from build123d import *

# Parameters (mm, degrees)
SKETCH1_R                   = 5.5
SKETCH1_W                   = 4
SKETCH1_H                   = 2
BOSS_EXTRUDE1_DEPTH         = 5
SKETCH2_R                   = 11.5
BOSS_EXTRUDE2_DEPTH         = 3
SKETCH3_R                   = 1.5
WHEEL_SCREWS_DEPTH          = 3
WHEEL_SCREW_PATTERN_COUNT   = 3
SKETCH5_R                   = 0.95
MOTOR_SCREW_HOLE_DEPTH      = 3
MOTOR_SCREW_HOLE_DEPTH_BACK = 8.474829283


with BuildPart() as part:
    # Sketch1 → Boss-Extrude1 (new body)
    with BuildSketch(Plane(origin=(0, 0, 0), x_dir=(1, 0, 0), z_dir=(0, 1, 0))):
        Circle(SKETCH1_R)
        with BuildLine():
            Line((-1.095, -1.025170717), (1.095, -1.025170717))
            ThreePointArc((1.095, -1.025170717), (0, 1.5), (-1.095, -1.025170717))
        make_face(mode=Mode.SUBTRACT)
        with Locations((0, -3.025170717)):
            Rectangle(SKETCH1_W, SKETCH1_H, mode=Mode.SUBTRACT)
    extrude(amount=BOSS_EXTRUDE1_DEPTH)

    # Sketch2 → Boss-Extrude2 (add)
    with BuildSketch(Plane(origin=(0, 5, 0), x_dir=(1, 0, 0), z_dir=(0, 1, 0))):
        Circle(SKETCH2_R)
    extrude(amount=BOSS_EXTRUDE2_DEPTH)

    # Sketch3 → wheel_screws (cut)
    with BuildSketch(Plane.XZ.offset(-5)):
        with Locations((0, -8.5)):
            Circle(SKETCH3_R)
    wheel_screws = extrude(amount=-WHEEL_SCREWS_DEPTH, mode=Mode.SUBTRACT)

    # wheel_screw_pattern: wheel_screws ×3 about axis
    wheel_screw_pattern_axis = Axis((0, 0, 0), (0, 1, 0))
    for i in range(1, WHEEL_SCREW_PATTERN_COUNT):
        add(wheel_screws.rotate(wheel_screw_pattern_axis, i * 360 / WHEEL_SCREW_PATTERN_COUNT), mode=Mode.SUBTRACT)

    # Sketch5 → motor_screw_hole (cut, two sides)
    with BuildSketch(Plane(origin=(0, 0, 4.025170717), x_dir=(-1, 0, 0), z_dir=(0, 0, -1))) as motor_screw_hole_sk:
        with Locations((0, 2.5)):
            Circle(SKETCH5_R)
    extrude(amount=MOTOR_SCREW_HOLE_DEPTH, mode=Mode.SUBTRACT)
    extrude(motor_screw_hole_sk.sketch, amount=-MOTOR_SCREW_HOLE_DEPTH_BACK, mode=Mode.SUBTRACT)


solid = part.part
Here's how the part is built. I have some questions about the finished solid (model axes, mm). A direction names the side the tool comes from. Coordinates: 2 decimals unless noted, no trailing zeros. Write each loop counter-clockwise with the first axis right and the second up, starting at its lowest first coordinate (ties: lowest second). Pieces come first, ordered by that corner, then holes.
Item 1: I want a section at D-D on z = 3.25. Write out the boundary of the cut face in (x, y).
Item 2: I want a section at A-A on z = 0. Write out the boundary of the cut face in (x, y).
Item 3: If I drill on line 1 (Z direction, x = 0, y = 3.7); line 2 (Z direction, x = 0, y = 7.2); line 3 (X direction, y = 6, z = 4.5), over which ranges is the centre line in solid material (lowest first)?
Item 4: Will these pins go through, and if not, where does the flat tip stop? pin 1 (1.6 mm diameter, centred on y = 3.5, z = 3, fed in from -X); pin 2 (2.5 mm diameter, centred on x = 0, y = 2.5, fed in from +Z); pin 3 (2 mm diameter, centred on y = 6, z = 9, fed in from +X).
Item 5: I want a section at B-B on x = 0. Write out the boundary of the cut face in (y, z), and give its area (3 significant figures).
Item 6: If we mould it in two halves opening along Z, with no side actions, what happens to faces 4 (the cylindrical face through (0, 6, -10)), 5 (the cylindrical face through (-1.5, 6.5, -11.4)), 6 (the flat face through (5, 5, -3))? For each: +Z half, -Z half, draft (parallel to the pull), parting line (faces both ways), or undercut.
Item 7: I want a section at C-C on x = -6.75. Write out the boundary of the cut face in (y, z).
Item 8: On a 3-axis mill with a long thin cutter (end or side, diameter ignored), from which of +Z, -Z, +X, -X, +Y, -Y can I reach the whole of each face in a straight line? I mean faces 1 (the flat face through (-1, 2, 2.025)), 2 (the flat face through (1.1, 0, -1.3)), 3 (the cylindrical face through (0.124, 3.442, 4.752)). Say none if no direction works.
Findings below:
1. outline: (-11.03, 5) - (-8.48, 5) - (-8.48, 8) - (-11.03, 8) - close; (-6.24, 5) - (-4.44, 5) - (-4.44, 0) - (-2, 0) - (-2, 5) - (2, 5) - (2, 0) - (4.44, 0) - (4.44, 5) - (6.24, 5) - (6.24, 8) - (-6.24, 8) - close; (8.48, 5) - (11.03, 5) - (11.03, 8) - (8.48, 8) - close
2. outline: (-11.5, 5) - (-5.5, 5) - (-5.5, 0) - (-1.5, 0) - (-1.5, 5) - (1.5, 5) - (1.5, 0) - (5.5, 0) - (5.5, 5) - (11.5, 5) - (11.5, 8) - (-11.5, 8) - close
3. line 1: z = -5.5 to -1.5, 1.03 to 2.03, 4.03 to 5.5
3. line 2: z = -11.5 to -10, -7 to 11.5
3. line 3: x = -10.58 to -8.84, -5.88 to 5.88, 8.84 to 10.58
4. pin 1: stops at x = -5.04
4. pin 2: stops at z = 5.5
4. pin 3: stops at x = 8.26
5. outline: (0, -5.5) - (5, -5.5) - (5, -7) - (8, -7) - (8, 11.5) - (5, 11.5) - (5, 5.5) - (3.45, 5.5) - (3.45, 4.03) - (5, 4.03) - (5, 2.03) - (3.45, 2.03) - (3.45, 1.03) - (5, 1.03) - (5, -1.5) - (0, -1.5) - close; (0, 1.03) - (1.55, 1.03) - (1.55, 2.03) - (0, 2.03) - close; (0, 4.03) - (1.55, 4.03) - (1.55, 5.5) - (0, 5.5) - close; (5, -11.5) - (8, -11.5) - (8, -10) - (5, -10) - close
5. area: 87.7 mm2
6. face 4: undercut
6. face 5: parting line
6. face 6: draft
7. outline: (5, -9.31) - (8, -9.31) - (8, 2.88) - (5, 2.88) - close; (5, 5.62) - (8, 5.62) - (8, 9.31) - (5, 9.31) - close
8. face 1: -Y
8. face 2: +Z, -Z, +X, -X, -Y
8. face 3: +Z
